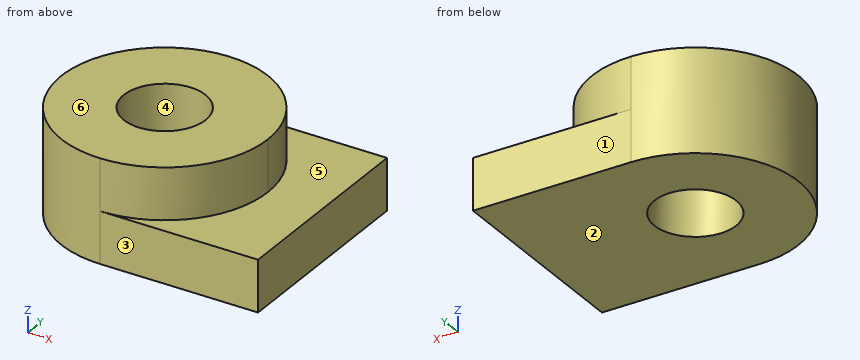
from build123d import *

# Parameters (mm, degrees)
F0_R     = 19.861396
F1_DEPTH = 50
F2_DEPTH = 25


with BuildPart() as f1:
    # F0 (on Top) → F1 (new body)
    with BuildSketch(Plane.XY):
        with BuildLine():
            ThreePointArc((0, -50.148256), (35.460172, -35.460172), (50.148256, 0))
            ThreePointArc((50.148256, 0), (35.460172, 35.460172), (0, 50.148256))
            ThreePointArc((0, 50.148256), (-50.148256, 0), (0, -50.148256))
        make_face()
        Circle(F0_R, mode=Mode.SUBTRACT)
    extrude(amount=F1_DEPTH)

    # F0 (on Top) → F2 (join)
    with BuildSketch(Plane.XY):
        with BuildLine():
            ThreePointArc((0, -50.148256), (35.460172, -35.460172), (50.148256, 0))
            ThreePointArc((50.148256, 0), (35.460172, 35.460172), (0, 50.148256))
            ThreePointArc((0, 50.148256), (-50.148256, 0), (0, -50.148256))
        make_face()
        Circle(F0_R, mode=Mode.SUBTRACT)
        with BuildLine():
            ThreePointArc((0, 50.148256), (35.460172, 35.460172), (50.148256, 0))
            ThreePointArc((50.148256, 0), (35.460172, -35.460172), (0, -50.148256))
            Line((0, -50.148256), (76.60187, -50.148256))
            Line((76.60187, -50.148256), (76.60187, 50.148256))
            Line((76.60187, 50.148256), (0, 50.148256))
        make_face()
    extrude(amount=F2_DEPTH)


solid = f1.part
Can you work these out from the model? Positions are in its coordinate system, mm. Face numbers are marked on the shaded views. A direction names the side the tool comes from. Coordinates: 2 decimals unless noted, no trailing zeros. Write each loop counter-clockwise with the first axis right and the second up, starting at its lowest first coordinate (ties: lowest second). Pieces come first, ordered by that corner, then holes. Notation, with made-up numbers: (59, 43) -> (116, 43) arc R19 cw to (116, 77) -> close; hole circle Ø6 at (6, -14). An arc over 180 degrees is marked (long way). Write each question's results on one line, items separated by ' | '. Start each with the question number.
Q1. Imagine slicing it at C-C (y = 38.5). Write out the boundary of the cut face in (x, z).
Q2. On a 3-axis mill with a long thin cutter (end or side, diameter ignored), from which of +Z, -Z, +X, -X, +Y, -Y can I reach the whole of each face in a straight line? I mean the marked faces 5 and 6. Say none if no direction works.
Q3. Imagine slicing it at B-B (z = 13). Write out the boundary of the cut face in (x, y), then the cut area to 3 significant figures.
Q4. If I drill on probe 1 along Z at (x, y) = (69, 17); probe 2 along Y at (x, z) = (14.5, 16.5); probe 3 along X at (y, z) = (10, 29), over which ranges is the centre line in solid material (lowest first)?
Q5. We'd pull the mould along Y, two halves only. Please class the marked faces 1, 2, 3 and 4: +Y half, -Y half, draft (parallel to the pull), parting line (faces both ways), or undercut.
Q6. Imagine slicing it at D-D (x = 38.5). Write out the boundary of the cut face in (y, z), then the cut area to 3 significant figures.
Q7. I'm going to push flat-ended pins straight in: pin 1 (2 mm diameter, centred on x = -1.5, z = 40, fed in from +Y); pin 2 (4 mm diameter, centred on x = 47.5, y = -24, fed in from +Z); pin 3 (1 mm diameter, centred on x = -20.5, z = 20, fed in from -Y). Where does each tip first touch, or does it pass through?
Taken from the geometry:
1) outline: (-32.13, 0) -> (76.6, 0) -> (76.6, 25) -> (32.13, 25) -> (32.13, 50) -> (-32.13, 50) -> close
2) face 5: +Z, +X | face 6: +Z, +X, -X, +Y, -Y
3) outline: (0, -50.15) -> (76.6, -50.15) -> (76.6, 50.15) -> (0, 50.15) arc R50.15 ccw to start; hole circle Ø39.72 at (0, 0) | area: 10,400 mm^2
4) probe 1: z = 0 to 25 | probe 2: y = -50.15 to -13.57, 13.57 to 50.15 | probe 3: x = -49.14 to -17.16, 17.16 to 49.14
5) face 1: +Y half | face 2: draft | face 3: -Y half | face 4: undercut
6) outline: (-50.15, 0) -> (50.15, 0) -> (50.15, 25) -> (32.13, 25) -> (32.13, 50) -> (-32.13, 50) -> (-32.13, 25) -> (-50.15, 25) -> close | area: 4,110 mm^2
7) pin 1: stops at y = 50.15 | pin 2: stops at z = 25 | pin 3: stops at y = -45.99
